Part model, mm, in its own coordinate system. Round coordinates to 2 decimals unless told otherwise and drop trailing zeros. Write each loop counter-clockwise with the first axis right and the second up, starting at its lowest first coordinate (ties: lowest second). Pieces come first, ordered by that corner, then holes. Notation, with made-up numbers: M 15,19 L 68,19 A17 ccw 68,30 Z; hole C 62.5,-0.5 d4. An arc over 180 degrees is marked long. Answer as a JSON object with one key per item and string values. Group by question number.
1. Band-saw the part on B-B, the plane z = 14.5. Write the cut outline in (x, y), plus the area to 3 significant figures.
2. Band-saw the part on C-C, the plane x = 4. Write the cut outline in (y, z).
3. Drill centre lines: line 1 (Z direction, x = 0, y = 2.25); line 2 (Z direction, x = 1, y = 2.75). Where is each one in solid material? Low to high. Write a range as from..to.
4. Band-saw the part on D-D, the plane y = 2.5. Count the separate pieces of the cut face and the enclosed holes in it, plus the area to 3 significant figures.
5. Band-saw the part on A-A, the plane x = 0. Write the cut outline in (y, z), plus the area to 3 significant figures.
6. Two-plate mould, pull along X, no slides. Class faces 1 (the face through (16.25, 3.45, -0.05)), 2 (the face through (-8, 0, -8)), 3 (the face through (13.887, 3.451, 10.648)): +X half, -X half, draft (parallel to the pull), parting line (faces both ways), or undercut.
Autodesk Inventor part; units mm, degrees
ref_plane "YZ Plane" through (0, 0, 0) normal (1, 0, 0) x (0, 1, 0)
ref_plane "XZ Plane" through (0, 0, 0) normal (0, 1, 0) x (-1, 0, 0)
ref_plane "XY Plane" through (0, 0, 0) normal (0, 0, 1) x (1, 0, 0)
sketch "Szkic1" plane through (0, 0, 0) normal (0, 1, 0) x (-1, 0, 0)
  circle A0 centre (0, 0) radius 10
  circle A1 centre (0, 0) radius 17.5
  line L0 (0, 17.5) -> (0, -17.5)
  line L1 (-17.5, 0) -> (17.5, 0)
  circle A2 centre (2.5, 2.5) radius 0.5
  circle A3 centre (2.5, -2.5) radius 0.5
  circle A4 centre (-2.5, 2.5) radius 0.5
  circle A5 centre (-2.5, -2.5) radius 0.5
  circle A6 centre (0, 15) radius 1.25
  circle A7 centre (0, -15) radius 1.25
  circle A8 centre (15, 0) radius 1.25
  circle A9 centre (-15, 0) radius 1.25
  line L2 (-2.5, -2.5) -> (-12.3744, -12.3744)
  line L3 (2.5, 2.5) -> (12.3744, 12.3744)
  line L4 (2.5, -2.5) -> (12.3744, -12.3744)
  line L5 (-2.5, 2.5) -> (-12.3744, 12.3744)
  circle A10 centre (10.6066, 10.6066) radius 1.25
  circle A11 centre (-10.6066, -10.6066) radius 1.25
  line L6 (-2.5, 2.5) -> (2.5, -2.5)
  line L7 (2.5, 2.5) -> (-2.5, -2.5)
  circle A12 centre (-10.6066, 10.6066) radius 1.25
  circle A13 centre (10.6066, -10.6066) radius 1.25
  dimension "d1" = 35
  dimension "d0" = 20
  dimension "d2" = 1
  dimension "d3" = 5
  dimension "d4" = 5
  dimension "d5" = 30
  dimension "d6" = 2.5
  dimension "d7" = 30
  dimension "d8" = 2.5
  dimension "d9" = 2.5
  dimension "d11" = 21.2132
extrude "Wyciągnięcie proste2" add sketch "Szkic1" along normal blind 7 contours L1 A8 A1 L4 A13 A0 | A0 L3 A10 A1 L1 A8 | A0 L0 A6 A1 L3 A10 | L4 A13 A1 L0 A7 A0 | A0 L5 A12 A1 L0 A6 | L0 A7 A1 L2 A11 A0 | L1 A9 A1 L5 A12 A0 | A0 L2 A11 A1 L1 A9
properties part number "doormy gora"
Worked answers:
{
 "1": {"outline": "M -9.8,0 L -1.15,0 L -1.15,7 L -9.8,7 Z; M 1.15,0 L 9.8,0 L 9.8,7 L 1.15,7 Z", "area": "121 mm^2"},
 "2": {"outline": "M 0,-17.04 L 7,-17.04 L 7,-9.17 L 0,-9.17 Z; M 0,9.17 L 7,9.17 L 7,17.04 L 0,17.04 Z"},
 "3": {"line 1": "z = -17.5..-16.25, -13.75..-10, 10..13.75, 16.25..17.5", "line 2": "z = -17.47..-15.75, -14.25..-9.95, 9.95..14.25, 15.75..17.47"},
 "4": {"separate pieces": "1", "enclosed holes": "9", "area": "609 mm^2"},
 "5": {"outline": "M 0,-17.5 L 7,-17.5 L 7,-16.25 L 0,-16.25 Z; M 0,-13.75 L 7,-13.75 L 7,-10 L 0,-10 Z; M 0,10 L 7,10 L 7,13.75 L 0,13.75 Z; M 0,16.25 L 7,16.25 L 7,17.5 L 0,17.5 Z", "area": "70.0 mm^2"},
 "6": {"face 1": "undercut", "face 2": "draft", "face 3": "parting line"}
}
